The listing builds one solid part. Answer for the finished solid, in the listing's coordinates (mm). Coordinates: 2 decimals unless noted, no trailing zeros. Use a Markdown table: item, result. Add a question column.
Item 1: Flat-ended cylindrical pins translate along their axes: P1, Ø1.5, axis at x = -34, z = 2, coming from the +Y side; P2, Ø2.5, axis at x = -2, z = 2, coming from the -Y side; P3, Ø1.5, axis at x = 42.5, z = 2.5, coming from the -Y side; P4, Ø8, axis at x = 7, y = -38.5, coming from the -Z side. Find the tip coordinate at first contact, or state that the pin passes through.
Item 2: The mould has two halves that part along X. Classify faces 1 (the flat face through (-4.225, 37.325, 2.465)), 2 (the flat face through (16, 1, 5)): released by +X, released by -X, zero draft, split by the parting line, or undercut.
Item 3: Find the intervals of material crossed by line 1 along X through (y, z) = (-25.5, 1.75); line 2 along X through (y, z) = (-45, 4.1); line 3 along Y through (x, z) = (-27, 1.1), in increasing order.
Item 4: The part is cut by section A-A, the plane x = 3. State how many separate pieces and enclosed holes the cut face has, then the cut area to 3 significant figures.
from build123d import *

# Parameters (mm, degrees)
F0_R     = 80
F1_DEPTH = 5
F3_DEPTH = 10
F4_R     = 2.49999
F5_DEPTH = 25


# Not quite as in the source:
# - a fillet or chamfer is up to 0.001 mm smaller than in the source, because OpenCascade refuses the exact size


with BuildPart() as f1:
    # F0 (on Top) → F1 (new body)
    with BuildSketch(Plane.XY):
        Circle(F0_R)
    extrude(amount=F1_DEPTH)

    # F2 (on Top) → F3 (cut)
    with BuildSketch(Plane.XY):
        Polygon((0, 50), (-25, 25), (-8.3333333333, 25), align=None)
        Polygon((-50, 0), (-16.6666666667, 0), (-20, 10), align=None)
        Polygon((-25, -25), (-12.5, -12.5), (-20, -10), align=None)
        Polygon((0, -25), (0, -16.6666666667), (-10, -20), (-8.3333333333, -25), align=None)
        Polygon((0, -50), (25, -25), (8.3333333333, -25), align=None)
        Polygon((0, 25), (0, 16.6666666667), (10, 20), (8.3333333333, 25), align=None)
        Polygon((25, 25), (12.5, 12.5), (20, 10), align=None)
        Polygon((50, 0), (25, 0), (25, -8.3333333333), align=None)
    extrude(amount=F3_DEPTH, mode=Mode.SUBTRACT)

    # F4 (radius 2.5 in the source; OpenCascade refuses exactly that, so slightly less here)
    f4_edges = [f1.edges().sort_by_distance(p)[0] for p in [
        (-80, 0, 0),
        (-80, 0, 5),
    ]]
    fillet(f4_edges, radius=F4_R)

    # F2 (on Top) → F5 (cut)
    with BuildSketch(Plane.XY):
        Polygon((0, -7.5), (0, 0), (-7.5, -7.5), align=None)
        Polygon((-7.5, -7.5), (0, 0), (-7.5, 0), align=None)
        Polygon((-7.5, 0), (0, 0), (-7.5, 7.5), align=None)
        Polygon((-7.5, 7.5), (0, 0), (0, 7.5), align=None)
        Polygon((0, 7.5), (0, 0), (7.5, 7.5), align=None)
        Polygon((7.5, 7.5), (0, 0), (7.5, 0), align=None)
        Polygon((7.5, 0), (0, 0), (7.5, -7.5), align=None)
    extrude(amount=F5_DEPTH, mode=Mode.SUBTRACT)


solid = f1.part
Solution:
| question | item | result |
|---|---|---|
| 1 | P1 | stops at y = 72.73 |
| 1 | P2 | stops at y = -80 |
| 1 | P3 | stops at y = -68.24 |
| 1 | P4 | stops at z = 0 |
| 2 | face 1 | undercut |
| 2 | face 2 | zero draft |
| 3 | line 1 | x = -75.71 to 8.17, 24.5 to 75.71 |
| 3 | line 2 | x = -65.44 to 1.67, 5 to 65.44 |
| 3 | line 3 | y = -74.85 to 0, 7.67 to 74.85 |
| 4 | separate pieces | 4 |
| 4 | enclosed holes | 0 |
| 4 | area | 675 mm2 |
